Check sheet for the modelled part. Datum: model origin and axes. Units: mm. A direction names the side the tool comes from. Give positions to 0.01 mm unless a question says otherwise; leave off trailing zeros. Loops run counter-clockwise (first coordinate to the right, second up) from the corner with the lowest first, then second, coordinate; pieces in that order, holes last. Notation, with made-up numbers: (-21, 26.5) -> (-1, 26.5) arc R20 cw to (-1, 33.5) -> close; hole circle Ø4 at (-24, 16). An arc over 180 degrees is marked (long way). Write each question's results on one line, items separated by ' | '. Start each with the question number.
1. Cross-section at D-D on y = 12.5. Record the boundary of the cut face in (x, z), and give its area (3 significant figures).
2. Cross-section at B-B on z = -9.5. Record the boundary of the cut face in (x, y), and give its area (3 significant figures).
3. Material ranges on L1, parallel to Y at x = 36.85, z = -6; L2, parallel to Z at x = 27.5, y = 17.75; L3, parallel to X at y = 17.25, z = -10, recorded low to high. Write a range as from..to.
4. Gauge pin test, flat ends, axial feed: pin 1 Ø1.5 at (x, z) = (31.5, -8) entering from -Y; pin 2 Ø1.2 at (y, z) = (5.4, -20) entering from +X; pin 3 Ø1.5 at (y, z) = (14, -6.5) entering from +X. Record the tip position at first contact, or that the pin passes through.
5. Tool access check on faces 5 (the face through (38, 13.6, -4.8)), 6 (the face through (4.972, 4.424, -10.217)), 7 (the face through (20, 12, -30)), 8 (the face through (6, 10, -15)), 9 (the face through (31, 10, -15)). Record the directions out of +Z, -Z, +X, -X, +Y, -Y that give a thin tool (end or side, any length) a straight path to the whole face; none if there is none.
6. Cross-section at C-C on y = 5.4. Record the boundary of the cut face in (x, z), and give its area (3 significant figures).
7. Mould release check, pull along Y, two halves, no side actions. Record for faces 1 (the face through (7, 5, -20)), 2 (the face through (5, 4.8, -20.8)), 3 (the face through (37.4, 14.56, -18.52)), 4 (the face through (14.41, 4.93, -15.21)): +Y half, -Y half, draft (parallel to the pull), parting line (faces both ways), or undercut.
8. Cross-section at A-A on z = -12.5. Record the boundary of the cut face in (x, y), and give its area (3 significant figures).
from build123d import *

# Parameters (mm, degrees)
SKETCH_1_W          = 41
SKETCH_1_H          = 30
SKETCH_1_R          = 1.5
EXTRUDE_1_DEPTH     = 10
SKETCH_3_W          = 30
SKETCH_3_H          = 8
CUT_EXTRUDE_2_DEPTH = 3
SKETCH_4_R          = 1
CUT_EXTRUDE_3_DEPTH = 7
EXTRUDE_3_DEPTH     = 30
SKETCH_6_W          = 20
SKETCH_6_H          = 30
CUT_EXTRUDE_5_DEPTH = 10
SKETCH_2_R          = 1.5
CUT_EXTRUDE_1_DEPTH = 6
SKETCH_8_R          = 1.5
CUT_EXTRUDE_6_DEPTH = 55.240206489
CUT_EXTRUDE_7_DEPTH = 55.240206489


with BuildPart() as part:
    # Эскиз1 → Бобышка-Вытянуть1 (new body)
    with BuildSketch(Plane(origin=(0, 0, 0), x_dir=(1, 0, 0), z_dir=(0, 1, 0))):
        with Locations((20.5, 15)):
            Rectangle(SKETCH_1_W, SKETCH_1_H)
        with Locations(Location((36.949747468, 19.949747468, 0), (0, 0, 270))):
            Circle(SKETCH_1_R, mode=Mode.SUBTRACT)
        with Locations(Location((27.050252532, 19.949747468, 0), (0, 0, 270))):
            Circle(SKETCH_1_R, mode=Mode.SUBTRACT)
        with Locations(Location((36.949747468, 10.050252532, 0), (0, 0, 270))):
            Circle(SKETCH_1_R, mode=Mode.SUBTRACT)
        with Locations(Location((27.050252532, 10.050252532, 0), (0, 0, 270))):
            Circle(SKETCH_1_R, mode=Mode.SUBTRACT)
    extrude(amount=EXTRUDE_1_DEPTH)

    # Эскиз3 → Вырез-Вытянуть2 (cut)
    with BuildSketch(Plane.ZY):
        with Locations((-15, 6)):
            Rectangle(SKETCH_3_W, SKETCH_3_H)
    extrude(amount=-CUT_EXTRUDE_2_DEPTH, mode=Mode.SUBTRACT)

    # Эскиз4 → Вырез-Вытянуть3 (cut)
    with BuildSketch(Plane.ZY):
        with Locations((-20, 5.4)):
            Circle(SKETCH_4_R)
        with Locations((-10, 5.4)):
            Circle(SKETCH_4_R)
    extrude(amount=-CUT_EXTRUDE_3_DEPTH, mode=Mode.SUBTRACT)

    # Эскиз7 → Бобышка-Вытянуть3 (add)
    with BuildSketch(Plane(origin=(0, 0, -30), x_dir=(-1, 0, 0), z_dir=(0, 0, -1))):
        Polygon((-41, 10), (-41, 19), (-21, 19), (-9, 10), align=None)
    extrude(amount=-EXTRUDE_3_DEPTH)

    # Эскиз6 → Вырез-Вытянуть5 (cut)
    with BuildSketch(Plane.XZ):
        with Locations((31, -15)):
            Rectangle(SKETCH_6_W, SKETCH_6_H)
    extrude(amount=-CUT_EXTRUDE_5_DEPTH, mode=Mode.SUBTRACT)

    # Эскиз2 → Вырез-Вытянуть1 (cut)
    with BuildSketch(Plane(origin=(41, 0, 0), x_dir=(0, 0, -1), z_dir=(1, 0, 0))):
        with Locations((6, 14.5)):
            Circle(SKETCH_2_R)
        with Locations((24, 14.5)):
            Circle(SKETCH_2_R)
    extrude(amount=-CUT_EXTRUDE_1_DEPTH, mode=Mode.SUBTRACT)

    # Эскиз8 → Вырез-Вытянуть6 (cut, through all)
    with BuildSketch(Plane(origin=(0, 19, 0), x_dir=(1, 0, 0), z_dir=(0, 1, 0))):
        with Locations(Location((36.949747468, 19.949747468, 0), (0, 0, 270))):
            Circle(SKETCH_8_R)
        with Locations(Location((36.949747468, 10.050252532, 0), (0, 0, 270))):
            Circle(SKETCH_8_R)
        with Locations(Location((27.050252532, 10.050252532, 0), (0, 0, 270))):
            Circle(SKETCH_8_R)
        with Locations(Location((27.050252532, 19.949747468, 0), (0, 0, 270))):
            Circle(SKETCH_8_R)
    extrude(amount=-CUT_EXTRUDE_6_DEPTH, mode=Mode.SUBTRACT)

    # Эскиз9 → Вырез-Вытянуть7 (cut, through all)
    with BuildSketch(Plane(origin=(0, 0, -30), x_dir=(-1, 0, 0), z_dir=(0, 0, -1))):
        Polygon((-21, 10), (-21, 0), (-8, 0), align=None)
    extrude(amount=-CUT_EXTRUDE_7_DEPTH, mode=Mode.SUBTRACT)


solid = part.part
Geometry says:
1) outline: (12.33, -30) -> (41, -30) -> (41, 0) -> (12.33, 0) -> close; hole circle Ø3 at (27.05, -19.95); hole circle Ø3 at (27.05, -10.05); hole circle Ø3 at (36.95, -19.95); hole circle Ø3 at (36.95, -10.05) | area: 832 mm^2
2) outline: (0, 0) -> (8, 0) -> (21, 10) -> (25.65, 10) -> (25.65, 19) -> (21, 19) -> (9, 10) -> (3, 10) -> (3, 6.27) -> (7, 6.27) -> (7, 4.53) -> (3, 4.53) -> (3, 2) -> (0, 2) -> close; (28.45, 10) -> (35.55, 10) -> (35.55, 19) -> (28.45, 19) -> close; (38.35, 10) -> (41, 10) -> (41, 19) -> (38.35, 19) -> close | area: 298 mm^2
3) L1: 10..13, 16..19 | L2: -30..-21.38, -18.52..-11.48, -8.62..0 | L3: 18.67..25.55, 28.55..35.45, 38.45..41
4) pin 1: y = 10 | pin 2: x = 15.8 | pin 3: x = 35
5) face 5: +X | face 6: -X | face 7: -Z, +X, -X, +Y, -Y | face 8: +Z, -Z, -X, +Y | face 9: +Z, -Z, +X, -Y
6) outline: (3, -30) -> (15.02, -30) -> (15.02, 0) -> (3, 0) -> (3, -9) -> (7, -9) -> (7, -11) -> (3, -11) -> (3, -19) -> (7, -19) -> (7, -21) -> (3, -21) -> close | area: 345 mm^2
7) face 1: undercut | face 2: undercut | face 3: draft | face 4: -Y half
8) outline: (0, 0) -> (8, 0) -> (21, 10) -> (41, 10) -> (41, 19) -> (21, 19) -> (9, 10) -> (3, 10) -> (3, 2) -> (0, 2) -> close | area: 355 mm^2
